from build123d import *

# Parameters (mm, degrees)
F0_W     = 65
F0_H     = 65
F0_W_2   = 60
F0_H_2   = 60
F1_DEPTH = 24
F2_DEPTH = 21


with BuildPart() as f1:
    # F0 (on Front) → F1 (new body)
    with BuildSketch(Plane.XZ):
        with Locations((-4.1498354938, 0)):
            Rectangle(F0_W, F0_H)
        with Locations((-4.1498354938, 0)):
            Rectangle(F0_W_2, F0_H_2, mode=Mode.SUBTRACT)
        with Locations((-4.1498354938, 0)):
            Rectangle(F0_W_2, F0_H_2)
    extrude(amount=F1_DEPTH)

    # F0 (on Front) → F2 (cut)
    with BuildSketch(Plane.XZ):
        with Locations((-4.1498354938, 0)):
            Rectangle(F0_W_2, F0_H_2)
    extrude(amount=F2_DEPTH, mode=Mode.SUBTRACT)


solid = f1.part
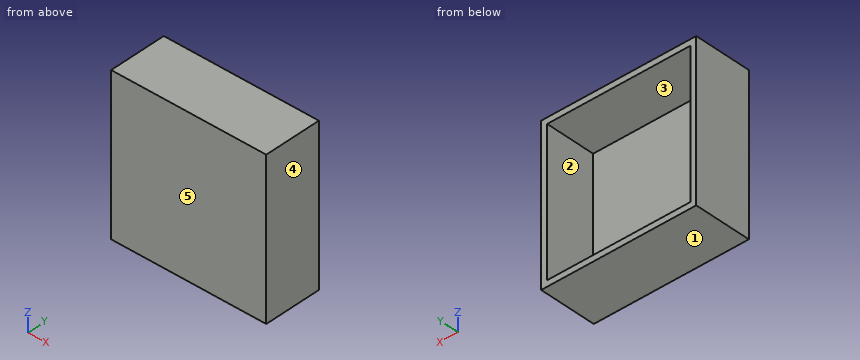
Design review of the part built by this model. Coordinates are the model's own, in mm. Face numbers are marked on the shaded views. A direction names the side the tool comes from. Coordinates: 2 decimals unless noted, no trailing zeros. Loops run counter-clockwise (first coordinate to the right, second up) from the corner with the lowest first, then second, coordinate; pieces in that order, holes last. Notation, with made-up numbers: (11.5, 13) -> (53.5, 13) arc R17 cw to (53.5, 26) -> close; hole circle Ø10 at (75, 68.5). An arc over 180 degrees is marked (long way). Use a Markdown table: item, result. Add a question column.
Item 1: Clearance check with a flat-ended pin moving along its axis: P1, Ø18, axis at x = 5.5, z = 6, coming from the +Y side. State where the tip first meets the part, or that it passes through.
Item 2: Machinability: for the marked faces 1 and 2, which of the approach directions +Z, -Z, +X, -X, +Y, -Y give a long, thin tool a straight path to every point of the face, cutting with its end or side? Answer none if there is none.
Item 3: We need section B-B, the plane x = -14. Write out the cut boundary in (y, z), and give its area (3 significant figures).
Item 4: The part is to be moulded in two halves that separate along X. For the marked faces 3, 4 and 5, say which applies: +X half, -X half, draft (parallel to the pull), parting line (faces both ways), or undercut.
Item 5: We need section A-A, the plane y = -13.5. Write out the cut boundary in (x, z).
Item 6: We need section C-C, the plane z = 8. Write out the cut boundary in (x, y), and give its area (3 significant figures).
Item 7: Wall thickness on L1, parallel to Z at x = 0, y = -20.75; L2, parallel to X at y = -13, z = 18; L3, parallel to Y at x = 7, z = 21: over which ranges is each line inside the solid? List them lowest first. Write a range as from..to.
Numbers:
| question | item | result |
|---|---|---|
| 1 | P1 | stops at y = -21 |
| 2 | face 1 | -Z, +X, -X, +Y, -Y |
| 2 | face 2 | +Y |
| 3 | outline | (-24, -32.5) -> (0, -32.5) -> (0, -30) -> (-21, -30) -> (-21, 30) -> (0, 30) -> (0, 32.5) -> (-24, 32.5) -> close |
| 3 | area | 300 mm^2 |
| 4 | face 3 | undercut |
| 4 | face 4 | +X half |
| 4 | face 5 | draft |
| 5 | outline | (-36.65, -32.5) -> (28.35, -32.5) -> (28.35, 32.5) -> (-36.65, 32.5) -> close; hole (-34.15, -30) -> (25.85, -30) -> (25.85, 30) -> (-34.15, 30) -> close |
| 6 | outline | (-36.65, -24) -> (28.35, -24) -> (28.35, 0) -> (25.85, 0) -> (25.85, -21) -> (-34.15, -21) -> (-34.15, 0) -> (-36.65, 0) -> close |
| 6 | area | 300 mm^2 |
| 7 | L1 | z = -32.5..-30, 30..32.5 |
| 7 | L2 | x = -36.65..-34.15, 25.85..28.35 |
| 7 | L3 | y = -24..-21 |
